Autodesk Inventor part; units mm, degrees
ref_plane "YZ Plane" through (0, 0, 0) normal (1, 0, 0) x (0, 1, 0)
ref_plane "XZ Plane" through (0, 0, 0) normal (0, 1, 0) x (-1, 0, 0)
ref_plane "XY Plane" through (0, 0, 0) normal (0, 0, 1) x (1, 0, 0)
sketch "Sketch1" plane through (0, 0, 0) normal (0, 1, 0) x (-1, 0, 0)
  circle A0 centre (0, 0) radius 9.271
  arc A1 (19.2643, -2.54) -> (19.2643, 2.54) centre (0, 0) ccw
  line L0 (19.431, 2.54) -> (14.351, 2.54)
  line L1 (14.351, 2.54) -> (14.351, -2.54)
  line L2 (14.351, -2.54) -> (19.431, -2.54)
  line L3 (19.431, -2.54) -> (19.431, 2.54)
  line L4 (19.431, 0) -> (0, 0) construction
  line L5 (-2.54, 19.431) -> (-2.54, 14.351)
  line L6 (-2.54, 14.351) -> (2.54, 14.351)
  line L7 (2.54, 14.351) -> (2.54, 19.431)
  line L8 (2.54, 19.431) -> (-2.54, 19.431)
  line L9 (-19.431, -2.54) -> (-14.351, -2.54)
  line L10 (-14.351, -2.54) -> (-14.351, 2.54)
  line L11 (-14.351, 2.54) -> (-19.431, 2.54)
  line L12 (-19.431, 2.54) -> (-19.431, -2.54)
  line L13 (2.54, -19.431) -> (2.54, -14.351)
  line L14 (2.54, -14.351) -> (-2.54, -14.351)
  line L15 (-2.54, -14.351) -> (-2.54, -19.431)
  line L16 (-2.54, -19.431) -> (2.54, -19.431)
  arc A2 (2.54, -19.2643) -> (13.1001, -14.351) centre (0, 0) ccw
  arc A3 (19.2643, 2.54) -> (2.54, 19.2643) centre (0, 0) ccw
  arc A4 (-19.2643, 2.54) -> (-19.2643, -2.54) centre (0, 0) ccw
  arc A5 (-19.2643, -2.54) -> (-2.54, -19.2643) centre (0, 0) ccw
  arc A6 (2.54, 19.2643) -> (-2.54, 19.2643) centre (0, 0) ccw
  arc A7 (-2.54, 19.2643) -> (-19.2643, 2.54) centre (0, 0) ccw
  arc A8 (13.1001, -14.351) -> (19.2643, -2.54) centre (0, 0) ccw
  arc A9 (-2.54, -19.2643) -> (2.54, -19.2643) centre (0, 0) ccw
  point P0 (0, 19.431)
  point P1 (-19.431, 0)
  point P2 (0, -19.431)
  dimension "d0" = 18.542
  dimension "d1" = 38.862
  dimension "d2" = 5.08
  dimension "d3" = 5.08
  dimension "d6" = 360
extrude "Extrusion1" add sketch "Sketch1" along normal blind 5.08 contours A8 A2 L13 L14 L15 A5 L9 L10 L11 A7 L5 L6 L7 A3 L0 L1 L2
properties part number "MarkerRing" material "Wood (Birch)"
Here's how the part is built. I have some questions about the finished solid (model axes, mm). A direction names the side the tool comes from. Coordinates: 2 decimals unless noted, no trailing zeros. Write each loop counter-clockwise with the first axis right and the second up, starting at its lowest first coordinate (ties: lowest second). Pieces come first, ordered by that corner, then holes. Notation, with made-up numbers: (-24, 18) -> (-9, 18) arc R16 ccw to (-9, 39) -> close; hole circle Ø5 at (85, 51.25). An arc over 180 degrees is marked (long way). Use a Markdown table: item, result. Add a question column.
(1) We'd pull the mould along Z, two halves only. Please class faces 1 (the cylindrical face through (13.87, 2.5, 13.61)), 2 (the flat face through (17, 3, -2.54)), 3 (the flat face through (2.54, 3, -17)), 4 (the cylindrical face through (-8.272, 2.504, -17.582)): +Z half, -Z half, draft (parallel to the pull), parting line (faces both ways), or undercut.
(2) If we section it at D-D, the plane z = -13: Write out the boundary of the cut face in (x, y), and give its area (3 significant figures).
(3) I'm going to push flat-ended pins straight in: P1, Ø2.5, axis at y = 2.5, z = 16.5, coming from the +X side; P2, Ø2.5, axis at y = 1.5, z = -18, coming from the -X side; P3, Ø1.5, axis at x = -7.5, z = 5, coming from the +Y side; P4, Ø15, axis at x = 0, z = 0, coming from the +Y side. Where does each tip first touch, or does it pass through?
(4) Please list where these lines run through material, in increasing order: line 1 (Z direction, x = 0, y = 1.4); line 2 (Z direction, x = -16, y = 3.45); line 3 (X direction, y = 3.95, z = -6.5).
(5) If we section it at C-C, the plane y = 0.5: Write out the boundary of the cut face in (x, z), and give its area (3 significant figures).
(6) If we section it at B-B, the plane z = 0: Write out the boundary of the cut face in (x, y), and give its area (3 significant figures).
(7) For faces 5 (the flat face through (-2.54, 3, -17)), 6 (the flat face through (-17, 3, 2.54)), 7 (the flat face through (17, 3, 2.54)), 8 (the flat face through (0, 3, 14.351)), which set-ups out of +Z, -Z, +X, -X, +Y, -Y let a thin tool reach every point of the face, with its end or its side?
(8) If we section it at A-A, the plane x = 0: Write out the boundary of the cut face in (y, z).
Outcome:
| question | item | result |
|---|---|---|
| 1 | face 1 | +Z half |
| 1 | face 2 | undercut |
| 1 | face 3 | draft |
| 1 | face 4 | -Z half |
| 2 | outline | (-14.44, 0) -> (14.44, 0) -> (14.44, 5.08) -> (-14.44, 5.08) -> close |
| 2 | area | 147 mm^2 |
| 3 | P1 | stops at x = 12.04 |
| 3 | P2 | stops at x = -9.85 |
| 3 | P3 | stops at y = 5.08 |
| 3 | P4 | passes through |
| 4 | line 1 | z = -14.35 to -9.27, 9.27 to 14.35 |
| 4 | line 2 | z = -11.03 to -2.54, 2.54 to 11.03 |
| 4 | line 3 | x = -18.31 to -6.61, 6.61 to 18.31 |
| 5 | outline | (-19.26, -2.54) arc R19.43 ccw to (-13.1, -14.35) arc R19.43 ccw to (-2.54, -19.26) -> (-2.54, -14.35) -> (2.54, -14.35) -> (2.54, -19.26) arc R19.43 ccw to (19.26, -2.54) -> (14.35, -2.54) -> (14.35, 2.54) -> (19.26, 2.54) arc R19.43 ccw to (2.54, 19.26) -> (2.54, 14.35) -> (-2.54, 14.35) -> (-2.54, 19.26) arc R19.43 ccw to (-19.26, 2.54) -> (-14.35, 2.54) -> (-14.35, -2.54) -> close; hole circle Ø18.54 at (0, 0) |
| 5 | area | 814 mm^2 |
| 6 | outline | (-14.35, 0) -> (-9.27, 0) -> (-9.27, 5.08) -> (-14.35, 5.08) -> close; (9.27, 0) -> (14.35, 0) -> (14.35, 5.08) -> (9.27, 5.08) -> close |
| 6 | area | 51.6 mm^2 |
| 7 | face 5 | -Z, +Y, -Y |
| 7 | face 6 | -X, +Y, -Y |
| 7 | face 7 | +X, +Y, -Y |
| 7 | face 8 | +Z, +Y, -Y |
| 8 | outline | (0, -14.35) -> (5.08, -14.35) -> (5.08, -9.27) -> (0, -9.27) -> close; (0, 9.27) -> (5.08, 9.27) -> (5.08, 14.35) -> (0, 14.35) -> close |
